Check sheet for the drawn part. Datum: minimum x, y, z corner. Units: mm. Give positions to 0.01 mm unless a question says otherwise; leave off trailing zeros. Order: outer loops, then holes, each group sorted by start corner. A loop starts at its lowest first (then second) coordinate and runs counter-clockwise, first axis right, second up.
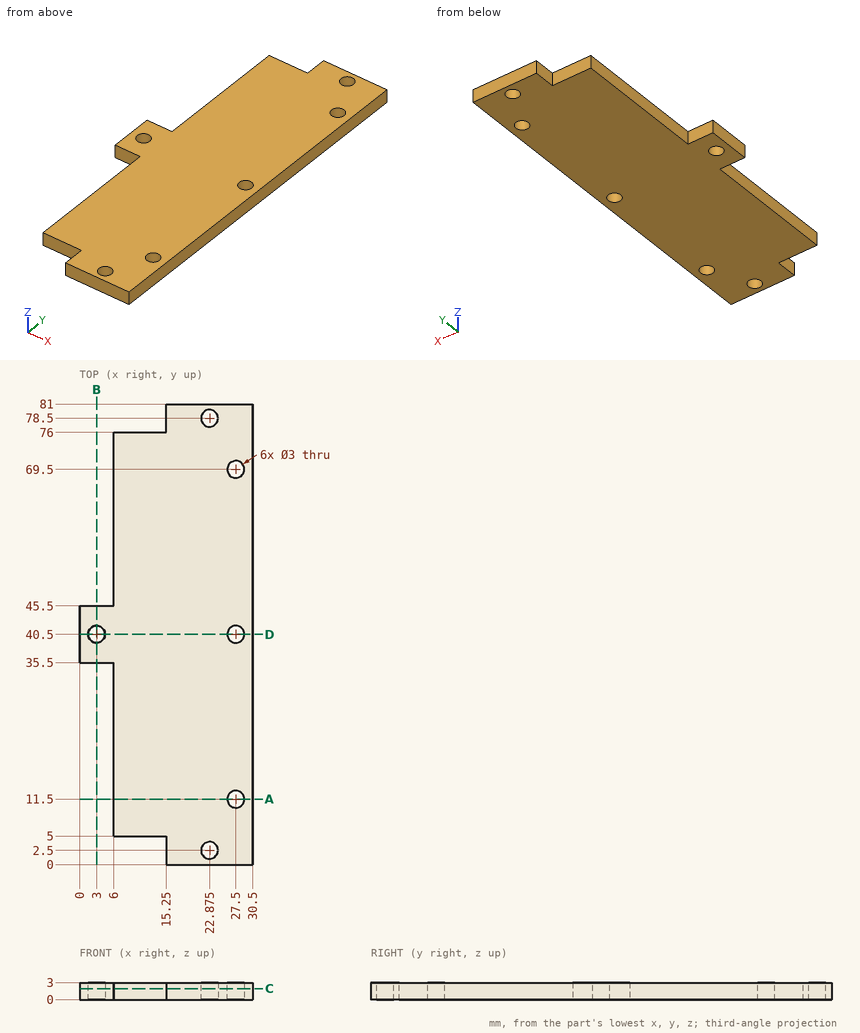
Item 1: Sectioned sample at B-B (x = 3). Enter the section's corners in (y, z), and give its area (3 significant figures).
Reported:
outline: (35.5, 0) - (39, 0) - (39, 3) - (35.5, 3) - close; (42, 0) - (45.5, 0) - (45.5, 3) - (42, 3) - close
area: 21.0 mm2
Item 2: Scan lines: L1, parallel to Y at x = 27.5, z = 1.6; L2, parallel to X at y = 69.5, z = 0.8; L3, parallel to X at y = 6.5, z = 1.8. Record each from-to range of solid material in increasing order.
Reported:
L1: y = 0 to 10, 13 to 39, 42 to 68, 71 to 81
L2: x = 6 to 26, 29 to 30.5
L3: x = 6 to 30.5
Item 3: Sectioned sample at D-D (y = 40.5). Enter the section's corners in (x, z), and give its area (3 significant figures).
Reported:
outline: (0, 0) - (1.5, 0) - (1.5, 3) - (0, 3) - close; (4.5, 0) - (26, 0) - (26, 3) - (4.5, 3) - close; (29, 0) - (30.5, 0) - (30.5, 3) - (29, 3) - close
area: 73.5 mm2
Item 4: Gauge pin test, flat ends, axial feed: pin 1 (0.9 mm diameter, centred on x = 10.5, z = 2, fed in from +Y); pin 2 (2.5 mm diameter, centred on x = 27.5, y = 69.5, fed in from +Z); pin 3 (0.9 mm diameter, centred on x = 12, z = 1, fed in from -Y); pin 4 (0.9 mm diameter, centred on x = 2, z = 1.5, fed in from -Y). Record the tip position at first contact, or that the pin passes through.
Reported:
pin 1: stops at y = 76
pin 2: passes through
pin 3: stops at y = 5
pin 4: stops at y = 35.5
Item 5: Sectioned sample at A-A (y = 11.5). Enter the section's corners in (x, z), and give its area (3 significant figures).
Reported:
outline: (6, 0) - (26, 0) - (26, 3) - (6, 3) - close; (29, 0) - (30.5, 0) - (30.5, 3) - (29, 3) - close
area: 64.5 mm2
Item 6: Sectioned sample at C-C (z = 1.95). Enter the section's corners in (x, y) (3 decimals).
Reported:
outline: (0, 35.5) - (6, 35.5) - (6, 5) - (15.25, 5) - (15.25, 0) - (30.5, 0) - (30.5, 81) - (15.25, 81) - (15.25, 76) - (6, 76) - (6, 45.5) - (0, 45.5) - close; hole circle Ø3 at (3, 40.5); hole circle Ø3 at (22.875, 2.5); hole circle Ø3 at (22.875, 78.5); hole circle Ø3 at (27.5, 11.5); hole circle Ø3 at (27.5, 40.5); hole circle Ø3 at (27.5, 69.5)
